Can you work these out from the model? Positions are in its coordinate system, mm. Coordinates: 2 decimals unless noted, no trailing zeros. Order: outer loops, then holes, each group sorted by start corner. A loop starts at its lowest first (then second) coordinate and runs counter-clockwise, first axis right, second up.
```python
from build123d import *

# Parameters (mm, degrees)
SKETCH1_W           = 210
SKETCH1_H           = 133
BOSS_EXTRUDE1_DEPTH = 6
CHAMFER1_SIZE       = 6


with BuildPart() as part:
    # Sketch1 → Boss-Extrude1 (new body)
    with BuildSketch(Plane(origin=(0, 0, 0), x_dir=(1, 0, 0), z_dir=(0, 1, 0))):
        Rectangle(SKETCH1_W, SKETCH1_H)
    extrude(amount=BOSS_EXTRUDE1_DEPTH)

    # Chamfer1
    chamfer1_edges = [part.edges().sort_by_distance(p)[0] for p in [
        (105, 0, 0),
        (-105, 0, 0),
    ]]
    chamfer(chamfer1_edges, length=CHAMFER1_SIZE - 0.0001)  # a hair under: the kernel refuses the full size


solid = part.part
```
1. I'm going to push a flat-ended pin straight in: pin 1 (1 mm diameter, centred on y = 4.5, z = -24.5, fed in from -X). Where does the tip first touch, or does it pass through?
Completed:
pin 1: stops at x = -104
2. Please list where these lines run through material, in increasing order: probe 1 along X at (y, z) = (1.75, -23); probe 2 along X at (y, z) = (5, 58).
Completed:
probe 1: x = -100.75 to 100.75
probe 2: x = -104 to 104
3. Imagine slicing it at B-B on y = 1.5. Please give me the cut outline in (x, z).
Completed:
outline: (-100.5, -66.5) - (100.5, -66.5) - (100.5, 66.5) - (-100.5, 66.5) - close
4. Thinking about a two-plate mould opening in X: for faces 1 (the flat face through (102, 3, 1)), 2 (the flat face through (-1, 3, 66.5)), 3 (the flat face through (-102, 3, 1)), which applies, pulls with the +X half, pulls with the -X half, needs draft (parallel to the pull), parting line crosses it, or undercut?
Completed:
face 1: pulls with the +X half
face 2: needs draft
face 3: pulls with the -X half
